```python
from build123d import *

# Parameters (mm, degrees)
F1_ANGLE_BACK = 45
F1_ANGLE      = 90
F2_R          = 2.5
F3_DEPTH      = 2
F4_R          = 6


with BuildPart() as f1:
    # F0 (on Right) → F1 (revolve)
    with BuildSketch(Plane.YZ, mode=Mode.PRIVATE) as f1_sk:
        with BuildLine():
            Line((65, 19), (65, 0))
            Line((65, 0), (67, 0))
            Line((67, 0), (67, 20))
            ThreePointArc((67, 20), (62, 25), (57, 20))
            Line((57, 20), (57, 0))
            Line((57, 0), (59, 0))
            Line((59, 0), (59, 19))
            Line((59, 19), (62, 22))
            Line((62, 22), (65, 19))
        make_face()
    revolve(f1_sk.sketch.rotate(Axis((0, 0, 11), (0, 0, 1)), -F1_ANGLE_BACK), axis=Axis((0, 0, 11), (0, 0, 1)), revolution_arc=F1_ANGLE)

    # F2 (on face) → F3 (join)
    with BuildSketch(Plane(origin=(0, 0, 0), x_dir=(1, 0, 0), z_dir=(0, 0, -1))):
        with BuildLine():
            ThreePointArc((0, -67), (-25.6397899685, -61.8999286783), (-47.3761543395, -47.3761543395))
            Line((-47.3761543395, -47.3761543395), (-47.3761543395, -67))
            Line((-47.3761543395, -67), (0, -67))
        make_face()
        with Locations((-40.8761543395, -60.5)):
            Circle(F2_R, mode=Mode.SUBTRACT)
        with BuildLine():
            ThreePointArc((47.3761543395, -47.3761543395), (25.6397899685, -61.8999286783), (0, -67))
            Line((0, -67), (47.3761543395, -67))
            Line((47.3761543395, -67), (47.3761543395, -47.3761543395))
        make_face()
        with Locations((40.8761543395, -60.5)):
            Circle(F2_R, mode=Mode.SUBTRACT)
    extrude(amount=-F3_DEPTH)

    # F4
    f4_edges = [f1.edges().sort_by_distance(p)[0] for p in [
        (-47.376154, 67, 1),
        (47.376154, 67, 1),
    ]]
    fillet(f4_edges, radius=F4_R)


solid = f1.part
```
Geometry check sheet. Reference: the model listing, model coordinates, mm. A direction names the side the tool comes from. Coordinates: 2 decimals unless noted, no trailing zeros. Order: outer loops, then holes, each group sorted by start corner. A loop starts at its lowest first (then second) coordinate and runs counter-clockwise, first axis right, second up.
Item 1: Scan lines: line 1 along X through (y, z) = (60.5, 1.2); line 2 along X through (y, z) = (50.5, 9.5); line 3 along Y through (x, z) = (0, 24). Record each from-to range of solid material in increasing order.
Item 2: Section check A-A (z = 7.75). Enter the section's corners in (x, y), plus the area to 3 significant figures.
Item 3: Mould release check, pull along Y, two halves, no side actions. Record for faces 1 (the conical face through (0.684, 62.184, 21.812)), 2 (the cylindrical face through (-45.57, 65.29, 1.01)), 3 (the flat face through (-46.1, 46.1, 12.7)): released by +Y, released by -Y, zero draft, split by the parting line, or undercut.
Item 4: Depth check by flat-ended pin: pin 1 (1 mm diameter, centred on x = -23.5, y = 62.5, fed in from +Z); pin 2 (8 mm diameter, centred on x = -40.88, y = 60.5, fed in from +Z); pin 3 (6 mm diameter, centred on y = 56.5, z = 21.5, fed in from +X). Enter the tip coordinate at first touch or a pass-through.
Item 5: Tool access check on faces 4 (the flat face through (36, 61, 2)), 5 (the cylindrical face through (0.737, 66.996, 11.126)), 6 (the cylindrical face through (0.649, 58.996, 9.633)), 7 (the flat face through (-36, 62, 2)). Record the directions out of +Z, -Z, +X, -X, +Y, -Y that give a thin tool (end or side, any length) a straight path to the whole face; none if there is none.
Check sheet entries:
1. line 1: x = -47.38 to -43.38, -38.38 to -23.76, 23.76 to 38.38, 43.38 to 47.38
1. line 2: x = -44.03 to -40.92, -30.51 to -26.43, 26.43 to 30.51, 40.92 to 44.03
1. line 3: y = 59 to 65
2. outline: (-47.38, 47.38) - (-45.96, 45.96) arc R65 cw to (45.96, 45.96) - (47.38, 47.38) arc R67 ccw to start; (-41.72, 41.72) - (-40.31, 40.31) arc R57 cw to (40.31, 40.31) - (41.72, 41.72) arc R59 ccw to start
2. area: 390 mm2
3. face 1: undercut
3. face 2: released by +Y
3. face 3: released by -Y
4. pin 1: stops at z = 22.6
4. pin 2: stops at z = 2
4. pin 3: stops at x = 40.12
5. face 4: +Z, +X, +Y
5. face 5: +Z, +Y
5. face 6: -Z
5. face 7: +Z, -X, +Y
